from build123d import *

# Parameters (mm, degrees)
ESQUISSE1_W                                        = 33
ESQUISSE1_H                                        = 33
BOSS_EXTRU_1_DEPTH                                 = 13
ESQUISSE3_R                                        = 2
ESQUISSE3_W                                        = 2.1
ESQUISSE3_H                                        = 2.8
ENL_V_MAT_EXTRU_1_DEPTH                            = 14
ESQUISSE4_W                                        = 11.606208868
ESQUISSE4_H                                        = 11.606208868
ESQUISSE4_R                                        = 2
ENL_V_MAT_EXTRU_2_DEPTH                            = 12.5
ESQUISSE2_R                                        = 1.2
ENL_V_MAT_EXTRU_3_DEPTH                            = 14
ESQUISSE5_W                                        = 20.32
ESQUISSE5_H                                        = 20.32
ENL_V_MAT_EXTRU_5_DEPTH                            = 10.5
ESQUISSE8_R                                        = 7.5
BOSS_EXTRU_4_DEPTH                                 = 13
CHAMBRAGE_POUR_VIS_T_TE_RONDE_BOMB_E_M_D           = 3.4
CHAMBRAGE_POUR_VIS_T_TE_RONDE_BOMB_E_M_CBORE_D     = 7
CHAMBRAGE_POUR_VIS_T_TE_RONDE_BOMB_E_M_CBORE_DEPTH = 2.4


with BuildPart() as part:
    # Esquisse1 → Boss.-Extru.1 (new body)
    with BuildSketch(Plane.XY):
        Rectangle(ESQUISSE1_W, ESQUISSE1_H)
    extrude(amount=BOSS_EXTRU_1_DEPTH)

    # Esquisse3 → Enlèv. mat.-Extru.1 (cut, through all)
    with BuildSketch(Plane.XY.offset(13)):
        with Locations((0.25, 0)):
            Circle(ESQUISSE3_R)
        with Locations((-2.97, 0)):
            Rectangle(ESQUISSE3_W, ESQUISSE3_H)
    extrude(amount=-ENL_V_MAT_EXTRU_1_DEPTH, mode=Mode.SUBTRACT)

    # Esquisse4 → Enlèv. mat.-Extru.2 (cut)
    with BuildSketch(Plane.XY.offset(13)):
        Rectangle(ESQUISSE4_W, ESQUISSE4_H)
        with Locations((0.25, 0)):
            Circle(ESQUISSE4_R, mode=Mode.SUBTRACT)
    extrude(amount=-ENL_V_MAT_EXTRU_2_DEPTH, mode=Mode.SUBTRACT)

    # Esquisse2 → Enlèv. mat.-Extru.3 (cut, through all)
    with BuildSketch(Plane.XY.offset(13)):
        with BuildLine():
            Line((7.62, 8.82), (-7.62, 8.82))
            ThreePointArc((-7.62, 8.82), (-8.82, 7.62), (-7.62, 6.42))
            Line((-7.62, 6.42), (7.62, 6.42))
            ThreePointArc((7.62, 6.42), (8.82, 7.62), (7.62, 8.82))
        make_face()
        with Locations((7.62, -7.62)):
            Circle(ESQUISSE2_R)
        with Locations((-7.62, -7.62)):
            Circle(ESQUISSE2_R)
    extrude(amount=-ENL_V_MAT_EXTRU_3_DEPTH, mode=Mode.SUBTRACT)

    # Esquisse5 → Enlèv. mat.-Extru.5 (cut)
    with BuildSketch(Plane.XY.offset(13)):
        Rectangle(ESQUISSE5_W, ESQUISSE5_H)
    extrude(amount=-ENL_V_MAT_EXTRU_5_DEPTH, mode=Mode.SUBTRACT)

    # Esquisse8 → Boss.-Extru.4 (add)
    with BuildSketch(Plane(origin=(0, 0, 0), x_dir=(-1, 0, 0), z_dir=(0, 0, -1))):
        with BuildLine():
            Line((19.228652316, -14.943489853), (19.228652316, 5.056510147))
            ThreePointArc((19.228652316, 5.056510147), (17.862916767, 5.087541175), (16.5, 5.180570213))
            Line((16.5, 5.180570213), (16.5, -14.869082996))
            ThreePointArc((16.5, -14.869082996), (17.863819007, -14.924884682), (19.228652316, -14.943489853))
        make_face()
        with BuildLine():
            ThreePointArc((-4.37758657, 16.5), (-9.179371873, 25.268372883), (-10.841194523, 35.126356986))
            Line((-10.841194523, 35.126356986), (-30.841194523, 35.126356986))
            ThreePointArc((-30.841194523, 35.126356986), (-27.117424712, 16.178251365), (-16.5, 0.048543968))
            Line((-16.5, 0.048543968), (-16.5, 16.5))
            Line((-16.5, 16.5), (-4.37758657, 16.5))
        make_face()
        with Locations((-19.609840661, 25.370666938)):
            Circle(ESQUISSE8_R, mode=Mode.SUBTRACT)
    extrude(amount=-BOSS_EXTRU_4_DEPTH)

    # Chambrage pour vis à tête ronde bombée M31 (through all)
    with Locations(Plane(origin=(-13.5, 13.5, 13), x_dir=(1, 0, 0), z_dir=(0, 0, 1))):
        with Locations((0, 0), (27, 0)):
            CounterBoreHole(CHAMBRAGE_POUR_VIS_T_TE_RONDE_BOMB_E_M_D / 2, CHAMBRAGE_POUR_VIS_T_TE_RONDE_BOMB_E_M_CBORE_D / 2, CHAMBRAGE_POUR_VIS_T_TE_RONDE_BOMB_E_M_CBORE_DEPTH)


solid = part.part
CAD build for the part. Positions are in the model's coordinates, mm. A direction names the side the tool comes from. Give positions to 0.01 mm unless a question says otherwise; leave off trailing zeros. Loops run counter-clockwise (first coordinate to the right, second up) from the corner with the lowest first, then second, coordinate; pieces in that order, holes last. Notation, with made-up numbers: M -15.5,71.25 L 25.5,71.25 A15 ccw 25.5,89.25 Z; hole C -37.75,-26.75 d5. An arc over 180 degrees is marked long. Answer in a Markdown table with one row per item. Add a question column.
Item 1: Band-saw the part on B-B on x = -13.5. Give the cut face in (y, z), then the cut area to 3 significant figures.
Item 2: Drop flat-ended pins along their axis: P1, Ø5, axis at x = 22, z = 10, coming from the -Y side; P2, Ø3, axis at x = 0.25, y = 0, coming from the +Z side; P3, Ø1.8, axis at y = -16, z = 8, coming from the -X side; P4, Ø8, axis at x = 10, y = -7, coming from the +Z side. Give the stop position or say it passes through.
Item 3: Tool access for faces 4 (the face through (-6, 16.5, 6)), 5 (the face through (0, -5.803, 2)), 6 (the face through (-8.82, 7.65, 1.27)): list every direction of +Z, -Z, +X, -X, +Y, -Y with a clear straight run to the whole face (end or side of a thin tool).
Item 4: Probe probe 1 along Y at (x, z) = (-0.5, 2); probe 2 along Y at (x, z) = (2.5, 11); probe 3 along X at (y, z) = (-3, 10.75). List the from-to ranges inside material, lowest first.
Item 5: Band-saw the part on D-D on z = 4.25. Give the cut face in (x, y).
Item 6: Band-saw the part on C-C on y = 29.5. Give the cut face in (x, z).
Item 7: Mould opens along X. For faces 1 (the face through (-19.229, -5, 6)), 2 (the face through (21, 35.126, 6)), 3 (the face through (6.42, -7.57, 1.27)) say: +X half, -X half, draft (parallel to the pull), parting line (faces both ways), or undercut.
Item 8: Band-saw the part on A-A on y = -7.62. Give the cut face in (x, z).
Reply:
| question | item | result |
|---|---|---|
| 1 | outline | M -16.5,0 L 11.8,0 L 11.8,10.6 L 10,10.6 L 10,13 L -16.5,13 Z; M 15.2,0 L 16.5,0 L 16.5,10.6 L 15.2,10.6 Z |
| 1 | area | 377 mm^2 |
| 2 | P1 | stops at y = 3.39 |
| 2 | P2 | passes through |
| 2 | P3 | stops at x = -16.5 |
| 2 | P4 | stops at z = 13 |
| 3 | face 4 | +Z, -Z, -X, +Y |
| 3 | face 5 | +Z |
| 3 | face 6 | +Z, -Z |
| 4 | probe 1 | y = -16.5 to -5.8, 5.8 to 6.42, 8.82 to 16.5 |
| 4 | probe 2 | y = -16.5 to -10.16, 10.16 to 16.5 |
| 4 | probe 3 | x = -19.23 to -10.16, 10.16 to 16.5 |
| 5 | outline | M -19.23,-14.94 A50.07 ccw -16.5,-14.87 L -16.5,-16.5 L 16.5,-16.5 L 16.5,0.05 A50.07 ccw 30.84,35.13 L 10.84,35.13 A30.07 cw 4.38,16.5 L -16.5,16.5 L -16.5,5.18 A30.07 cw -19.23,5.06 Z; hole C -13.5,13.5 d3.4; hole M -10.16,-10.16 L 10.16,-10.16 L 10.16,10.16 L -10.16,10.16 Z; hole C 13.5,13.5 d3.4; hole C 19.61,25.37 d15 |
| 6 | outline | M 10.31,0 L 13.35,0 L 13.35,13 L 10.31,13 Z; M 25.87,0 L 30.52,0 L 30.52,13 L 25.87,13 Z |
| 7 | face 1 | -X half |
| 7 | face 2 | draft |
| 7 | face 3 | undercut |
| 8 | outline | M -19.23,0 L -8.82,0 L -8.82,2.5 L -10.16,2.5 L -10.16,13 L -19.23,13 Z; M -6.42,0 L 6.42,0 L 6.42,2.5 L -6.42,2.5 Z; M 8.82,0 L 16.5,0 L 16.5,13 L 10.16,13 L 10.16,2.5 L 8.82,2.5 Z |
